```python
from build123d import *

# Parameters (mm, degrees)
EXTRUDE1_DEPTH      = 5.7
SKETCH2_OUTSIDE_W   = 73.328
SKETCH2_OUTSIDE_H   = 73.328
SKETCH2_OUTSIDE_R   = 7.5
CUT_EXTRUDE1_DEPTH  = 12.4
CUT_EXTRUDE1_TAPER  = 60
SKETCH5_R           = 5
CUT_EXTRUDE10_DEPTH = 12.4
SKETCH16_R          = 7.5
SKETCH16_RX         = 5
SKETCH16_RY         = 4.4
EXTRUDE2_DEPTH      = 11.4


with BuildPart() as part:
    # Sketch20 → Extrude1 (new body, symmetric)
    with BuildSketch(Plane.XY):
        Polygon((7.5, -4.330127019), (7.5, 4.330127019), (0, 8.660254038), (-7.5, 4.330127019), (-7.5, -4.330127019), (0, -8.660254038), align=None)
    extrude(amount=EXTRUDE1_DEPTH, both=True)

    # Sketch18 → Revolve1 (revolve)
    with BuildSketch(Plane(origin=(0, 0, 0), x_dir=(0, 0, -1), z_dir=(1, 0, 0))):
        with BuildLine():
            Line((5.7, 0), (5.7, 10.9))
            Line((5.7, 10.9), (4.2, 10.9))
            ThreePointArc((4.2, 10.9), (-0.760606441, 6.423589339), (-2.6, 0))
            Line((-2.6, 0), (5.7, 0))
        make_face()
    revolve(axis=Axis((0, 0, -5.7), (0, 0, 1)))

    # Sketch2 outside → Cut-Extrude1 (cut, through all)
    with BuildSketch(Plane.XY.offset(5.7)):
        Rectangle(SKETCH2_OUTSIDE_W, SKETCH2_OUTSIDE_H)
        Circle(SKETCH2_OUTSIDE_R, mode=Mode.SUBTRACT)
    extrude(amount=-CUT_EXTRUDE1_DEPTH, taper=CUT_EXTRUDE1_TAPER, mode=Mode.SUBTRACT)

    # Sketch5 → Cut-Extrude10 (cut, through all)
    with BuildSketch(Plane(origin=(0, 0, 5.7), x_dir=(-1, 0, 0), z_dir=(0, 0, -1))):
        Circle(SKETCH5_R)
    extrude(amount=CUT_EXTRUDE10_DEPTH, mode=Mode.SUBTRACT)

    # Sketch16 → Extrude2 (add)
    with BuildSketch(Plane.XY.offset(5.7)):
        Circle(SKETCH16_R)
        with Locations(Location((0, 0), (0, 0, 90))):
            Ellipse(SKETCH16_RX, SKETCH16_RY, mode=Mode.SUBTRACT)
    extrude(amount=-EXTRUDE2_DEPTH)


solid = part.part
```
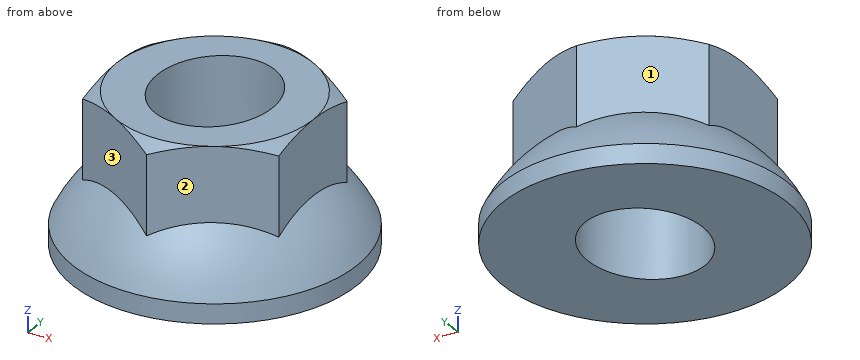
Check sheet for the modelled part. Datum: model origin and axes. Units: mm. Face numbers are marked on the shaded views. A direction names the side the tool comes from. Coordinates: 2 decimals unless noted, no trailing zeros. Write each loop counter-clockwise with the first axis right and the second up, starting at its lowest first coordinate (ties: lowest second). Pieces come first, ordered by that corner, then holes. Notation, with made-up numbers: (7.25, 40) -> (55.25, 40) arc R36 cw to (55.25, 75) -> close; hole circle Ø10 at (38.25, 37.25). An arc over 180 degrees is marked (long way). Use a Markdown table: item, result.
1. Sectioned sample at B-B (x = 8.5). Enter the section's corners in (y, z), plus the area to 3 significant figures.
Reported:
| item | result |
|---|---|
| outline | (-6.82, -5.7) -> (6.82, -5.7) -> (6.82, -4.2) arc R8.66 ccw to (-6.82, -4.2) -> close |
| area | 52.1 mm2 |
2. Sectioned sample at A-A (x = -9). Enter the section's corners in (y, z).
Reported:
| item | result |
|---|---|
| outline | (-6.15, -5.7) -> (6.15, -5.7) -> (6.15, -4.2) arc R8.14 ccw to (-6.15, -4.2) -> close |
3. Scan lines: line 1 along Y through (x, z) = (-0.25, -2); line 2 along X through (y, z) = (1.5, 3); line 3 along X through (y, z) = (-2.25, -3). Record each from-to range of solid material in increasing order.
Reported:
| item | result |
|---|---|
| line 1 | y = -9.51 to -4.99, 4.99 to 9.51 |
| line 2 | x = -7.5 to -4.2, 4.2 to 7.5 |
| line 3 | x = -9.98 to -3.93, 3.93 to 9.98 |
4. Go/stop test with flat-tipped pins: pin 1 Ø3 at (y, z) = (-7.5, -4) entering from -X; pin 2 Ø2 at (x, z) = (-8, -4) entering from -Y; pin 3 Ø1.5 at (x, z) = (-8.5, -2.5) entering from -Y. Record where each tip stops, or that it passes through.
Reported:
| item | result |
|---|---|
| pin 1 | stops at x = -9.09 |
| pin 2 | stops at y = -8.34 |
| pin 3 | stops at y = -6.44 |
5. Tool access check on the marked faces 1, 2 and 3. Record the directions out of +Z, -Z, +X, -X, +Y, -Y that give a thin tool (end or side, any length) a straight path to the whole face; none if there is none.
Reported:
| item | result |
|---|---|
| face 1 | +Z, -X, +Y |
| face 2 | +Z, +X, -Y |
| face 3 | +Z, -X, -Y |
